from build123d import *

# Parameters (mm, degrees)
ESBO_O1_W                = 14
ESBO_O1_H                = 12
RESSALTO_EXTRUS_O1_DEPTH = 2
ESBO_O2_W                = 2.5
ESBO_O2_H                = 13.9
RESSALTO_EXTRUS_O2_DEPTH = 9
ESBO_O3_W                = 2.5
ESBO_O3_H                = 8
RESSALTO_EXTRUS_O3_DEPTH = 9
RESSALTO_EXTRUS_O4_START = -15
ESBO_O4_R                = 3.5
RESSALTO_EXTRUS_O4_DEPTH = 2
ESBO_O6_R                = 1.75
CORTE_EXTRUS_O1_DEPTH    = 2.5
FILETE1_R                = 0.5


with BuildPart() as part:
    # Esboço1 → Ressalto-extrusão1 (new body)
    with BuildSketch(Plane(origin=(0, 0, 0), x_dir=(1, 0, 0), z_dir=(0, 1, 0))):
        with BuildLine():
            Line((116, -21), (117, -8))
            Line((117, -8), (117, 8))
            Line((117, 8), (116, 21))
            Line((116, 21), (102, 21))
            Line((102, 21), (102, 29))
            ThreePointArc((102, 29), (99.363961031, 35.363961031), (93, 38))
            Line((93, 38), (0, 38))
            Line((0, 38), (0, -38))
            Line((0, -38), (93, -38))
            ThreePointArc((93, -38), (99.363961031, -35.363961031), (102, -29))
            Line((102, -29), (102, -21))
            Line((102, -21), (116, -21))
        make_face()
        with Locations((60, -27.8)):
            Rectangle(ESBO_O1_W, ESBO_O1_H, mode=Mode.SUBTRACT)
        with Locations((60, 27.8)):
            Rectangle(ESBO_O1_W, ESBO_O1_H, mode=Mode.SUBTRACT)
    extrude(amount=RESSALTO_EXTRUS_O1_DEPTH)

    # Esboço2 → Ressalto-extrusão2 (add)
    with BuildSketch(Plane(origin=(0, 2, 0), x_dir=(1, 0, 0), z_dir=(0, 1, 0))):
        Polygon((111.5, 7.747296355), (109.530384494, 7.4), (107.446606362, 19.217693036), (109.416221868, 19.564989391), align=None)
        with Locations((114.75, 0)):
            Rectangle(ESBO_O2_W, ESBO_O2_H)
        Polygon((107.446606362, -19.217693036), (109.530384494, -7.4), (111.5, -7.747296355), (109.416221868, -19.564989391), align=None)
    extrude(amount=RESSALTO_EXTRUS_O2_DEPTH)

    # Esboço3 → Ressalto-extrusão3 (add)
    with BuildSketch(Plane(origin=(0, 2, 0), x_dir=(1, 0, 0), z_dir=(0, 1, 0))):
        with Locations((2.25, -11.5)):
            Rectangle(ESBO_O3_W, ESBO_O3_H)
        with Locations((2.25, 11.5)):
            Rectangle(ESBO_O3_W, ESBO_O3_H)
    extrude(amount=RESSALTO_EXTRUS_O3_DEPTH)

    # Esboço4 → Ressalto-extrusão4 (add)
    with BuildSketch(Plane.XY.offset(38).offset(RESSALTO_EXTRUS_O4_START)):
        Polygon((8.00982099, 2), (8.00982099, 19.434528411), (22.205610886, 19.434528411), (41.330494496, 2), align=None)
        with Locations((17.00982099, 10.717264205)):
            Circle(ESBO_O4_R, mode=Mode.SUBTRACT)
    ressalto_extrus_o4 = extrude(amount=RESSALTO_EXTRUS_O4_DEPTH)

    # Espelhar1: Ressalto-extrusão4 across plane
    add(ressalto_extrus_o4.mirror(Plane.XY))

    # Esboço6 → Corte-extrusão1 (cut)
    with BuildSketch(Plane.ZY.offset(-1)):
        with Locations((11.5, 7)):
            Circle(ESBO_O6_R)
    corte_extrus_o1 = extrude(amount=-CORTE_EXTRUS_O1_DEPTH, mode=Mode.SUBTRACT)

    # Espelhar2: Corte-extrusão1 across plane
    add(corte_extrus_o1.mirror(Plane.XY), mode=Mode.SUBTRACT)

    # Filete1
    filete1_edges = [part.edges().sort_by_distance(p)[0] for p in [
        (116, 6.5, 6.95),
        (116, 6.5, -6.95),
        (113.5, 6.5, -6.95),
        (113.5, 6.5, 6.95),
        (111.5, 6.5, -7.747296355),
        (109.416221868, 6.5, -19.564989391),
        (107.446606362, 6.5, -19.217693036),
        (109.530384494, 6.5, -7.4),
        (107.446606362, 6.5, 19.217693036),
        (109.416221868, 6.5, 19.564989391),
        (111.5, 6.5, 7.747296355),
        (109.530384494, 6.5, 7.4),
    ]]
    fillet(filete1_edges, radius=FILETE1_R)


solid = part.part
The model under review builds one solid part; all positions refer to its coordinate system, in mm. A direction names the side the tool comes from. Round coordinates to 2 decimals unless told otherwise and drop trailing zeros. Write each loop counter-clockwise with the first axis right and the second up, starting at its lowest first coordinate (ties: lowest second). Pieces come first, ordered by that corner, then holes. Notation, with made-up numbers: M 84.5,-21.75 L 141.5,-21.75 A32 ccw 141.5,10.25 Z; hole C 49.5,31 d10. An arc over 180 degrees is marked long. Use a Markdown table: item, result. Add a question column.
Q1. We need section C-C, the plane y = 15.5. State the section outline as (x, z) points, plus the area to 3 significant figures.
Q2. The part is to be moulded in two halves that separate along X. For faces 1 (the face through (1, 5, 11)), 2 (the face through (16.25, 7.3, 23.99)), 3 (the face through (3.5, 5, 11)), 4 (the face through (21, 9, 23)), say which applies: pulls with the +X half, pulls with the -X half, needs draft (parallel to the pull), parting line crosses it, or undercut.
Q3. To check wall thickness, follow line 1 (Z direction, x = 16, y = 17.5); line 2 (Y direction, x = 65.5, z = 8.5); line 3 (X direction, y = 8, z = 4.5). State the ranges of each line that lie inside material, in increasing order.
Q4. Insertion check: pin 1 (1.6 mm diameter, centred on y = 10, z = -23.5, fed in from -X); pin 2 (1.2 mm diameter, centred on x = 115, y = 5, fed in from -Z); pin 3 (12 mm diameter, centred on x = 77.5, z = 18.5, fed in from +Y); pin 4 (10 mm diameter, centred on x = 94.5, z = 12, fed in from -Y). Each pin has a flat end and moves straight along its axis. Give the tip position at first contact, or say it passes through.
Q5. We need section A-A, the plane x = 60. State the section outline as (y, z) points, plus the area to 3 significant figures.
Q6. Machinability: for faces 5 (the face through (110.47, 6.44, 13.58)), 6 (the face through (108.475, 6.437, 13.385)), 7 (the face through (2, 6, -15.5)), 8 (the face through (113.5, 6, 0)), which of the approach directions +Z, -Z, +X, -X, +Y, -Y give a long, thin tool a straight path to every point of the face, cutting with its end or side? Answer none if there is none.
Q7. We need section B-B, the plane z = -11.5. State the section outline as (x, y) points.
Findings below:
| question | item | result |
|---|---|---|
| 1 | outline | M 8.01,-25 L 26.52,-25 L 26.52,-23 L 8.01,-23 Z; M 8.01,23 L 26.52,23 L 26.52,25 L 8.01,25 Z |
| 1 | area | 74.0 mm² |
| 2 | face 1 | pulls with the -X half |
| 2 | face 2 | undercut |
| 2 | face 3 | undercut |
| 2 | face 4 | needs draft |
| 3 | line 1 | z = -25 to -23, 23 to 25 |
| 3 | line 2 | y = 0 to 2 |
| 3 | line 3 | x = 113.5 to 116 |
| 4 | pin 1 | stops at x = 8.01 |
| 4 | pin 2 | stops at z = -6.95 |
| 4 | pin 3 | stops at y = 2 |
| 4 | pin 4 | stops at y = 0 |
| 5 | outline | M 0,-38 L 2,-38 L 2,-33.8 L 0,-33.8 Z; M 0,-21.8 L 2,-21.8 L 2,21.8 L 0,21.8 Z; M 0,33.8 L 2,33.8 L 2,38 L 0,38 Z |
| 5 | area | 104 mm² |
| 6 | face 5 | +Z, +X, +Y |
| 6 | face 6 | +Y |
| 6 | face 7 | -Z, -X, +Y |
| 6 | face 8 | +Z, -Z, -X, +Y |
| 7 | outline | M 0,0 L 116.73,0 L 116.73,2 L 110.84,2 L 110.84,11 L 108.81,11 L 108.81,2 L 3.5,2 L 3.5,5.25 L 1,5.25 L 1,2 L 0,2 Z; M 1,8.75 L 3.5,8.75 L 3.5,11 L 1,11 Z |
